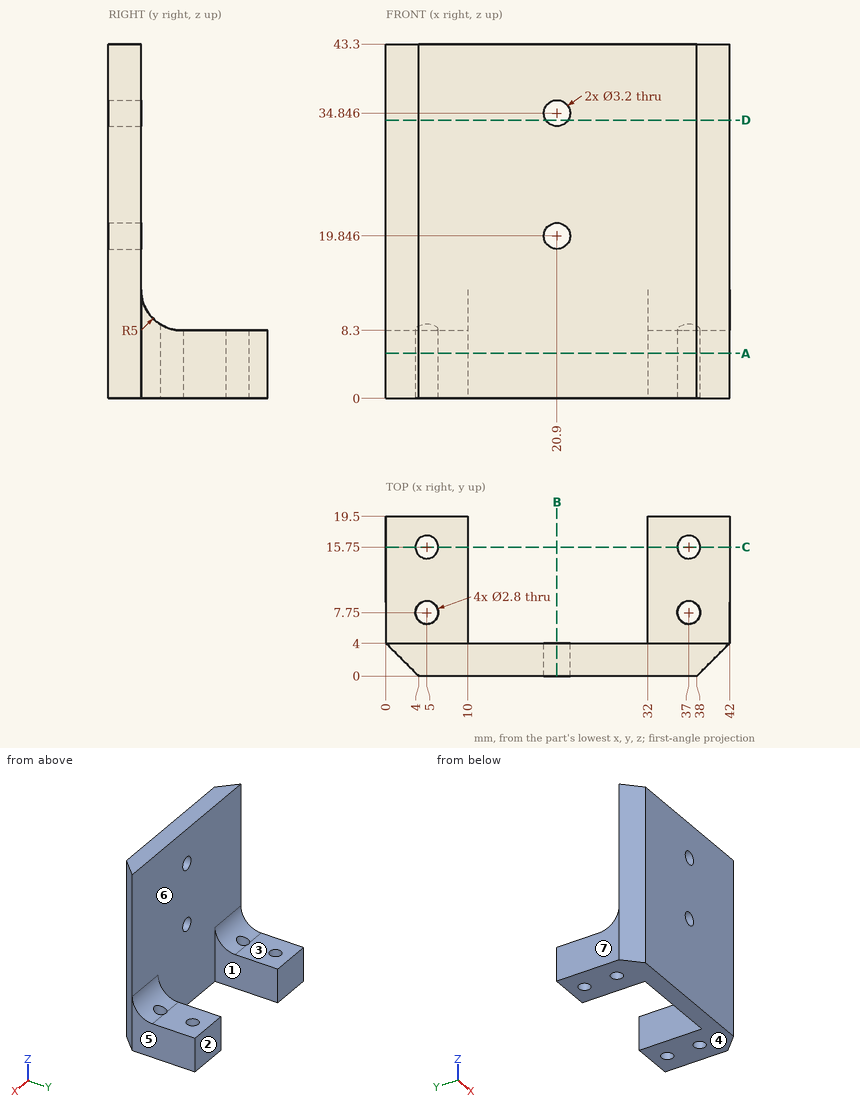
Geometry check sheet. Reference: drawing and pictorial views, mm from the part's lowest x, y, z. A direction names the side the tool comes from. Give positions to 0.01 mm unless a question says otherwise; leave off trailing zeros. Loops run counter-clockwise (first coordinate to the right, second up) from the corner with the lowest first, then second, coordinate; pieces in that order, holes last. Notation, with made-up numbers: (-37.5, 64.25) - (-30.5, 64.25) arc R13 ccw to (-30.5, 68.25) - close; hole circle Ø10 at (28, 35). An arc over 180 degrees is marked (long way). Use CSV: the item, a comma, the result in double quotes. Start each with the question number.
Q1. Section check A-A, the plane z = 5.5. Record the cut outline in (x, y), and give its area (3 significant figures).
Q2. Section check D-D, the plane z = 34. Record the cut outline in (x, y).
Q3. Go/stop test with flat-tipped pins: pin 1 Ø3 at (x, y) = (9, 10.5) entering from +Z; pin 2 Ø3 at (x, y) = (37, 7.75) entering from -Z; pin 3 Ø5 at (x, z) = (20.9, 19.85) entering from +Y. Record where each tip stops, or that it passes through.
Q4. Section check B-B, the plane x = 20.9. Record the cut outline in (y, z), and give its area (3 significant figures).
Q5. Access from +Z, -Z, +X, -X, +Y, -Y to the whole of each face (thin tool, end or side, straight path). Record for the marked faces 1, 2 and 3.
Q6. Section check C-C, the plane y = 15.75. Record the cut outline in (x, z).
Q7. Release check for a two-part mould opening along X. For the marked faces 4, 5, 6 and 7 record: +X half, -X half, draft (parallel to the pull), parting line (faces both ways), or undercut.
Q8. Scan lines: probe 1 along X at (y, z) = (7.75, 6); probe 2 along Y at (x, z) = (5, 6.5); probe 3 along Y at (x, z) = (10, 38.5). Record each from-to range of solid material in increasing order. Write a range as from..to.
Findings below:
1,outline,"(0, 4) - (4, 0) - (38, 0) - (42, 4) - (42, 19.5) - (32, 19.5) - (32, 4) - (10, 4) - (10, 19.5) - (0, 19.5) - close; hole circle Ø2.8 at (5, 7.75); hole circle Ø2.8 at (5, 15.75); hole circle Ø2.8 at (37, 7.75); hole circle Ø2.8 at (37, 15.75)"
1,area,"437 mm^2"
2,outline,"(0, 4) - (4, 0) - (19.54, 0) - (19.54, 4) - close; (22.26, 0) - (38, 0) - (42, 4) - (22.26, 4) - close"
3,pin 1,"stops at z = 8.3"
3,pin 2,"stops at z = 0"
3,pin 3,"stops at y = 4"
4,outline,"(0, 0) - (4, 0) - (4, 18.25) - (0, 18.25) - close; (0, 21.45) - (4, 21.45) - (4, 33.25) - (0, 33.25) - close; (0, 36.45) - (4, 36.45) - (4, 43.3) - (0, 43.3) - close"
4,area,"148 mm^2"
5,face 1,"+Z, -Z, +Y"
5,face 2,"+Z, -Z, +X, -X, +Y"
5,face 3,"+Z, +X, -X, +Y"
6,outline,"(0, 0) - (3.6, 0) - (3.6, 8.3) - (0, 8.3) - close; (6.4, 0) - (10, 0) - (10, 8.3) - (6.4, 8.3) - close; (32, 0) - (35.6, 0) - (35.6, 8.3) - (32, 8.3) - close; (38.4, 0) - (42, 0) - (42, 8.3) - (38.4, 8.3) - close"
7,face 4,"draft"
7,face 5,"+X half"
7,face 6,"undercut"
7,face 7,"-X half"
8,probe 1,"x = 0..3.6, 6.4..10, 32..35.6, 38.4..42"
8,probe 2,"y = 0..6.35, 9.15..14.35, 17.15..19.5"
8,probe 3,"y = 0..4"
